Could you check a few things on this model? Use its own coordinates, in mm. A direction names the side the tool comes from. Give positions to 0.01 mm unless a question says otherwise; leave off trailing zeros. Loops run counter-clockwise (first coordinate to the right, second up) from the corner with the lowest first, then second, coordinate; pieces in that order, holes last. Notation, with made-up numbers: (77, 84.25) - (121, 84.25) arc R10 cw to (121, 91.25) - close; hole circle Ø4 at (3, 22). An arc over 180 degrees is marked (long way). One line per item, written item: value. Start each with the question number.
Q1. I want a section at A-A (y = 48). Please give me the cut outline in (x, z).
Q2. If I drill on line 1 (Z direction, x = 35, y = 42); line 2 (Y direction, x = 43.5, z = 31.5); line 3 (X direction, y = 52, z = 4.5), over which ranges is the centre line in solid material (lowest first)? Write a range as from..to.
Q3. I want a section at D-D (y = 36.5). Please give me the cut outline in (x, z), then the cut area to 4 significant figures.
Q4. I want a section at C-C (x = 8). Please give me the cut outline in (y, z).
Q5. I'm going to push flat-ended pins straight in: P1, Ø5, axis at y = 37.5, z = 36.5, coming from the +X side; P2, Ø8, axis at x = 16, z = 30, coming from the -Y side; P3, Ø20, axis at x = 45.5, y = 44, coming from the +Z side; P4, Ø6, axis at x = 48.5, z = 44, coming from the +Y side. Where does each tip first touch, or does it pass through?
Q6. For faces 1 (the face through (40, 24, 40)), 2 (the face through (23, 8, 60)), which set-ups out of +Z, -Z, +X, -X, +Y, -Y let a thin tool reach every point of the face, with its end or its side?
Q7. I want a section at B-B (z = 44). Please give me the cut outline in (x, y), then the cut area to 3 significant figures.
```python
from build123d import *

# Parameters (mm, degrees)
CROQUIS1_W              = 60
CROQUIS1_H              = 60
SALIENTE_EXTRUIR1_DEPTH = 60
CROQUIS6_W              = 40
CROQUIS6_H              = 20
CORTAR_EXTRUIR2_DEPTH   = 40
CORTAR_EXTRUIR3_DEPTH   = 60
CORTAR_EXTRUIR4_DEPTH   = 20
CORTAR_EXTRUIR5_DEPTH   = 20


with BuildPart() as part:
    # Croquis1 → Saliente-Extruir1 (new body)
    with BuildSketch(Plane(origin=(0, 0, 0), x_dir=(1, 0, 0), z_dir=(0, 1, 0))):
        with Locations((30, -30)):
            Rectangle(CROQUIS1_W, CROQUIS1_H)
    extrude(amount=SALIENTE_EXTRUIR1_DEPTH)

    # Croquis6 → Cortar-Extruir2 (cut)
    with BuildSketch(Plane(origin=(0, 60, 0), x_dir=(1, 0, 0), z_dir=(0, 1, 0))):
        with Locations((40, -50)):
            Rectangle(CROQUIS6_W, CROQUIS6_H)
    extrude(amount=-CORTAR_EXTRUIR2_DEPTH, mode=Mode.SUBTRACT)

    # Croquis2 → Cortar-Extruir3 (cut)
    with BuildSketch(Plane.XY.offset(60)):
        Polygon((60, 60), (20, 60), (60, 20), align=None)
    extrude(amount=-CORTAR_EXTRUIR3_DEPTH, mode=Mode.SUBTRACT)

    # Croquis7 → Cortar-Extruir4 (cut)
    with BuildSketch(Plane.XY.offset(60)):
        Polygon((20, 20), (60, 0), (60, 20), align=None)
    extrude(amount=-CORTAR_EXTRUIR4_DEPTH, mode=Mode.SUBTRACT)

    # Croquis8 → Cortar-Extruir5 (cut)
    with BuildSketch(Plane(origin=(20, 0, 0), x_dir=(0, 0, -1), z_dir=(1, 0, 0))):
        Polygon((-40, 60), (-60, 20), (-60, 60), align=None)
    extrude(amount=-CORTAR_EXTRUIR5_DEPTH, mode=Mode.SUBTRACT)


solid = part.part
```
Worked answers:
1. outline: (0, 0) - (32, 0) - (32, 40) - (20, 40) - (20, 46) - (0, 46) - close
2. line 1: z = 0..40
2. line 2: y = 0..36.5
2. line 3: x = 0..28
3. outline: (0, 0) - (43.5, 0) - (43.5, 40) - (20, 40) - (20, 51.75) - (0, 51.75) - close
3. area: 1,975 mm²
4. outline: (0, 0) - (60, 0) - (60, 40) - (20, 60) - (0, 60) - close
5. P1: stops at x = 45
5. P2: stops at y = 0
5. P3: stops at z = 40
5. P4: stops at y = 7.25
6. face 1: +Z, +X, +Y
6. face 2: +Z, +X, -X, +Y, -Y
7. outline: (0, 0) - (60, 0) - (20, 20) - (20, 52) - (0, 52) - close
7. area: 1,440 mm²
